The listing builds one solid part. Answer for the finished solid, in the listing's coordinates (mm). Give positions to 0.01 mm unless a question says otherwise; leave off trailing zeros. Order: outer loops, then holes, each group sorted by start corner. A loop starts at its lowest first (then second) coordinate and runs counter-clockwise, first axis right, second up. Notation, with made-up numbers: M 77.5,60 L 93.5,60 A12 cw 93.5,65 Z; hole C 66,53.5 d7. An arc over 180 degrees is marked long. Answer as a JSON object with one key per item and string values. Group by question number.
```python
from build123d import *

# Parameters (mm, degrees)
SKETCH1_W                                      = 19.98
SKETCH1_H                                      = 128.4
BOSS_EXTRUDE1_DEPTH                            = 2.5
CUT_EXTRUDE1_DEPTH                             = 127.049239982
CUT_EXTRUDE2_DEPTH                             = 127.049239982
SKETCH4_W                                      = 3.9
SKETCH4_H                                      = 14.6
CUT_EXTRUDE3_DEPTH                             = 127.049239982
F_3_0_3_DIAMETER_HOLE1_D                       = 3
CSK_FOR_M2_5_FLAT_HEAD_MACHINE_SCREW1_AT_COUNT = 2
CSK_FOR_M2_5_FLAT_HEAD_MACHINE_SCREW1_AT_PITCH = 99.130249672
USB_DEPTH                                      = 127.049239982
SKETCH10_W                                     = 4
SKETCH10_H                                     = 4
MCXX_DEPTH                                     = 127.049239982
COPY_MMCX_1_COUNT                              = 3
COPY_MMCX_1_PITCH                              = 6
COPY_MMCX_2_COUNT                              = 2
COPY_MMCX_2_PITCH                              = 51
COPY_MMCX_2_COPY_1_SKETCH_W                    = 4
COPY_MMCX_2_COPY_1_SKETCH_H                    = 4
COPY_MMCX_2_COPY_1_DEPTH                       = 127.049239982
COPY_MMCX_2_COPY_2_SKETCH_W                    = 4
COPY_MMCX_2_COPY_2_SKETCH_H                    = 4
COPY_MMCX_2_COPY_2_DEPTH                       = 127.049239982
SKETCH12_R                                     = 3
SELECTOR_1_DEPTH                               = 127.049239982
LPATTERN3_COUNT                                = 3
LPATTERN3_PITCH                                = 11


with BuildPart() as part:
    # Sketch1 → Boss-Extrude1 (new body)
    with BuildSketch(Plane.XY.offset(2.5)):
        with Locations((2.54, 61.2)):
            Rectangle(SKETCH1_W, SKETCH1_H)
    extrude(amount=-BOSS_EXTRUDE1_DEPTH)

    # Sketch2 → Cut-Extrude1 (cut, through all)
    with BuildSketch(Plane.XY.offset(2.5)):
        with BuildLine():
            Line((2.445403852, 124.05), (-2.445403852, 124.05))
            ThreePointArc((-2.445403852, 124.05), (-2.95, 122.4), (-2.445403852, 120.75))
            Line((-2.445403852, 120.75), (2.445403852, 120.75))
            ThreePointArc((2.445403852, 120.75), (2.95, 122.4), (2.445403852, 124.05))
        make_face()
    extrude(amount=-CUT_EXTRUDE1_DEPTH, mode=Mode.SUBTRACT)

    # Sketch3 → Cut-Extrude2 (cut, through all)
    with BuildSketch(Plane.XY.offset(2.5)):
        with BuildLine():
            Line((7.525403852, 1.65), (2.634596148, 1.65))
            ThreePointArc((2.634596148, 1.65), (2.13, 0), (2.634596148, -1.65))
            Line((2.634596148, -1.65), (7.525403852, -1.65))
            ThreePointArc((7.525403852, -1.65), (8.03, 0), (7.525403852, 1.65))
        make_face()
    extrude(amount=-CUT_EXTRUDE2_DEPTH, mode=Mode.SUBTRACT)

    # Sketch4 → Cut-Extrude3 (cut, through all)
    with BuildSketch(Plane(origin=(0, 0, 0), x_dir=(-1, 0, 0), z_dir=(0, 0, -1))):
        with Locations((1.87, 8.5)):
            Rectangle(SKETCH4_W, SKETCH4_H)
    extrude(amount=-CUT_EXTRUDE3_DEPTH, mode=Mode.SUBTRACT)

    # Ø3.0 (3) Diameter Hole1 (through all)
    with Locations(Plane.XY.offset(2.5)):
        with Locations((-3.95, 119.1)):
            Hole(F_3_0_3_DIAMETER_HOLE1_D / 2)

    # Sketch7 → CSK for M2.5 Flat Head Machine Screw1 (revolve, cut)
    with BuildSketch(Plane(origin=(5.08, 11.7, 2.5), x_dir=(0, -1, 0), z_dir=(1, 0, 0))):
        Polygon((0, 0), (0, 2.5), (1.35, 2.5), (1.35, 1.5), (2.5, 0.35), (2.5, 0), align=None)
    csk_for_m2_5_flat_head_machine_screw1 = revolve(axis=Axis((5.08, 11.7, 8.85), (0, 0, -1)), mode=Mode.SUBTRACT)

    # CSK for M2.5 Flat Head Machine Screw1 at: CSK for M2.5 Flat Head Machine Screw1 ×2
    with Locations(*[Vector(-0.05124570972853528, 0.9986860754183062, 0) * (i * CSK_FOR_M2_5_FLAT_HEAD_MACHINE_SCREW1_AT_PITCH) for i in range(1, CSK_FOR_M2_5_FLAT_HEAD_MACHINE_SCREW1_AT_COUNT)]):
        add(csk_for_m2_5_flat_head_machine_screw1, mode=Mode.SUBTRACT)

    # Sketch9 → USB (cut, through all)
    with BuildSketch(Plane.XY.offset(2.5)):
        Polygon((-3.82, 19.95), (1.78, 19.95), (1.78, 32.45), (-3.82, 32.45), (-6.95, 32.45), (-6.95, 19.95), align=None)
    extrude(amount=-USB_DEPTH, mode=Mode.SUBTRACT)

    # Sketch10 → MCXX (cut, through all)
    with BuildSketch(Plane.XY.offset(2.5)):
        with Locations((-1.82, 35.2)):
            Rectangle(SKETCH10_W, SKETCH10_H)
    mcxx = extrude(amount=-MCXX_DEPTH, mode=Mode.SUBTRACT)

    # Copy MMCX 1: MCXX ×3
    with Locations(*[(0, i * COPY_MMCX_1_PITCH, 0) for i in range(1, COPY_MMCX_1_COUNT)]):
        add(mcxx, mode=Mode.SUBTRACT)

    # Copy MMCX 2: MCXX ×2
    with Locations(*[(0, i * COPY_MMCX_2_PITCH, 0) for i in range(1, COPY_MMCX_2_COUNT)]):
        add(mcxx, mode=Mode.SUBTRACT)

    # Copy MMCX 2 copy 1 sketch → Copy MMCX 2 copy 1 (cut, through all)
    with BuildSketch(Plane(origin=(0, 57, 2.5), x_dir=(1, 0, 0), z_dir=(0, 0, 1))):
        with Locations((-1.82, 35.2)):
            Rectangle(COPY_MMCX_2_COPY_1_SKETCH_W, COPY_MMCX_2_COPY_1_SKETCH_H)
    extrude(amount=-COPY_MMCX_2_COPY_1_DEPTH, mode=Mode.SUBTRACT)

    # Copy MMCX 2 copy 2 sketch → Copy MMCX 2 copy 2 (cut, through all)
    with BuildSketch(Plane(origin=(0, 63, 2.5), x_dir=(1, 0, 0), z_dir=(0, 0, 1))):
        with Locations((-1.82, 35.2)):
            Rectangle(COPY_MMCX_2_COPY_2_SKETCH_W, COPY_MMCX_2_COPY_2_SKETCH_H)
    extrude(amount=-COPY_MMCX_2_COPY_2_DEPTH, mode=Mode.SUBTRACT)

    # Sketch12 → Selector 1 (cut, through all)
    with BuildSketch(Plane.XY.offset(2.5)):
        with Locations((2.68, 55.2)):
            Circle(SKETCH12_R)
    selector_1 = extrude(amount=-SELECTOR_1_DEPTH, mode=Mode.SUBTRACT)

    # LPattern3: Selector 1 ×3
    with Locations(*[(0, i * LPATTERN3_PITCH, 0) for i in range(1, LPATTERN3_COUNT)]):
        add(selector_1, mode=Mode.SUBTRACT)


solid = part.part
```
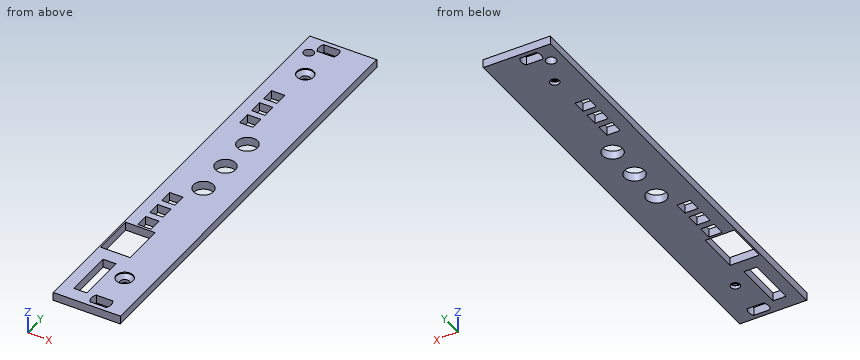
Item 1: Section A-A (y = 66.2) is taken. Determine the outline of the cut face in (x, z).
Item 2: Section C-C (z = 0.6) is taken. Count the separate pieces of the cut face and the enclosed holes in it, and give its area (3 significant figures).
Item 3: Section B-B (y = 7) is taken. Determine the outline of the cut face in (x, z).
Item 4: Section D-D (y = 110.7) is taken. Determine the outline of the cut face in (x, z), and give its area (3 significant figures).
Item 5: Consider probe 1 along Y at (x, z) = (7, 2); probe 2 along X at (y, z) = (110.7, 0.7); probe 3 along X at (y, z) = (100, 1.25). Determine where each line is inside the solid, lowest interval first. Write a range as from..to.
Item 6: A flat-ended cylindrical pin translates along its axis: P1, Ø10, axis at x = 1.5, y = 102.5, coming from the -Z side. Find the tip coordinate at first contact, or state that the pin passes through.
Values found:
{
 "1": {"outline": "M -7.45,0 L -0.32,0 L -0.32,2.5 L -7.45,2.5 Z; M 5.68,0 L 12.53,0 L 12.53,2.5 L 5.68,2.5 Z"},
 "2": {"separate pieces": "1", "enclosed holes": "16", "area": "2,160 mm^2"},
 "3": {"outline": "M -7.45,0 L -3.82,0 L -3.82,2.5 L -7.45,2.5 Z; M 0.08,0 L 12.53,0 L 12.53,2.5 L 0.08,2.5 Z"},
 "4": {"outline": "M -7.45,0 L -1.35,0 L -1.35,1 L -2.5,2.15 L -2.5,2.5 L -7.45,2.5 Z; M 1.35,0 L 12.53,0 L 12.53,2.5 L 2.5,2.5 L 2.5,2.15 L 1.35,1 Z", "area": "41.1 mm^2"},
 "5": {"probe 1": "y = -3..-1.65, 1.65..10.34, 13.06..125.4", "probe 2": "x = -7.45..-1.35, 1.35..12.53", "probe 3": "x = -7.45..-3.82, 0.18..12.53"},
 "6": {"P1": "stops at z = 0"}
}
